Autodesk Inventor part; units mm, degrees
ref_plane "YZ Plane" through (0, 0, 0) normal (1, 0, 0) x (0, 1, 0)
ref_plane "XZ Plane" through (0, 0, 0) normal (0, 1, 0) x (-1, 0, 0)
ref_plane "XY Plane" through (0, 0, 0) normal (0, 0, 1) x (1, 0, 0)
sketch "スケッチ1" plane through (0, 0, 0) normal (0, 0, 1) x (1, 0, 0)
  line L0 (2.75, 1.5877) -> (2.75, -1.5877)
  line L1 (2.75, -1.5877) -> (0, -3.1754)
  line L2 (0, -3.1754) -> (-2.75, -1.5877)
  line L3 (-2.75, -1.5877) -> (-2.75, 1.5877)
  line L4 (-2.75, 1.5877) -> (0, 3.1754)
  line L5 (0, 3.1754) -> (2.75, 1.5877)
  point P0 (0, 0)
  point P1 (0, 0)
  dimension "d0" = 5.5
extrude "押し出し1" add sketch "スケッチ1" along normal blind 24.5
sketch "スケッチ2" plane through (0, 0, 24.5) normal (0, 0, 1) x (1, 0, 0)
  point P0 (0, 0)
  point P1 (0, 0)
hole "穴1" at (0, 0, 24.5) direction (0, 0, -1) diameter 2.459 depth 6
mirror "ミラー1" about plane through (0, 0, 0) normal (0, 0, -1) of "押し出し1", "穴1"
properties part number "ASU-340" material "ステンレス鋼 AISI 304"
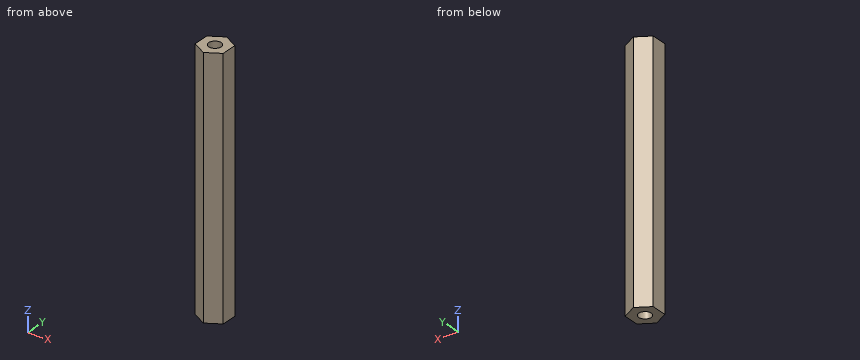
Geometry check sheet. Reference: the model listing, model coordinates, mm. Round coordinates to 2 decimals unless told otherwise and drop trailing zeros. Loops run counter-clockwise (first coordinate to the right, second up) from the corner with the lowest first, then second, coordinate; pieces in that order, holes last. Notation, with made-up numbers: (61, 81) - (120, 81) arc R16 cw to (120, 99) - close; hole circle Ø9 at (-9.5, 0). An arc over 180 degrees is marked (long way). Write item = value, one per line. Start each with the question number.
1. Depth check by flat-ended pin: pin 1 (1.2 mm diameter, centred on x = 0, y = 0.5, fed in from +Z); pin 2 (1.5 mm diameter, centred on x = -0.5, z = 3, fed in from -Y); pin 3 (1.2 mm diameter, centred on x = 0, y = -0.5, fed in from -Z). Enter the tip coordinate at first touch or a pass-through.
2. Section check D-D on y = 2.5. Enter the section's corners in (x, z).
3. Section check C-C on x = 0.8. Enter the section's corners in (y, z).
4. Section check B-B on z = 11. Enter the section's corners in (x, y), then the cut area to 3 significant figures.
5. Section check A-A on y = 0. Enter the section's corners in (x, z).
6. Thickness scan on line 1 (X direction, y = 0, z = 21.15); line 2 (Y direction, x = 0, z = -22.35); line 3 (Y direction, x = -0.75, z = 16). Record the ranges inside material, lowest first.
Working result:
q1.pin_1 = 18.5
q1.pin_2 = -3.18
q1.pin_3 = -18.5
q2.outline = (-1.17, -24.5) - (1.17, -24.5) - (1.17, 24.5) - (-1.17, 24.5) - close
q3.outline = (-2.71, -24.5) - (-0.93, -24.5) - (-0.93, -18.5) - (0.93, -18.5) - (0.93, -24.5) - (2.71, -24.5) - (2.71, 24.5) - (0.93, 24.5) - (0.93, 18.5) - (-0.93, 18.5) - (-0.93, 24.5) - (-2.71, 24.5) - close
q4.outline = (-2.75, -1.59) - (0, -3.18) - (2.75, -1.59) - (2.75, 1.59) - (0, 3.18) - (-2.75, 1.59) - close
q4.area = 26.2 mm^2
q5.outline = (-2.75, -24.5) - (-1.23, -24.5) - (-1.23, -18.5) - (1.23, -18.5) - (1.23, -24.5) - (2.75, -24.5) - (2.75, 24.5) - (1.23, 24.5) - (1.23, 18.5) - (-1.23, 18.5) - (-1.23, 24.5) - (-2.75, 24.5) - close
q6.line_1 = -2.75 to -1.23, 1.23 to 2.75
q6.line_2 = -3.18 to -1.23, 1.23 to 3.18
q6.line_3 = -2.74 to 2.74
